Check sheet for the modelled part. Datum: model origin and axes. Units: mm. Face numbers are marked on the shaded views. A direction names the side the tool comes from. Coordinates: 2 decimals unless noted, no trailing zeros. Loops run counter-clockwise (first coordinate to the right, second up) from the corner with the lowest first, then second, coordinate; pieces in that order, holes last.
```python
from build123d import *

# Parameters (mm, degrees)
SKETCH1_R           = 50
BOSS_EXTRUDE1_DEPTH = 35
SKETCH2_R           = 5
BOSS_EXTRUDE2_DEPTH = 45
FILLET1_R           = 10
SKETCH3_R           = 19.698674941
CUT_EXTRUDE1_DEPTH  = 5
SKETCH4_R           = 17.698674941
CUT_EXTRUDE2_DEPTH  = 1
SKETCH5_R           = 15.698674941
CUT_EXTRUDE3_DEPTH  = 1


with BuildPart() as part:
    # Sketch1 → Boss-Extrude1 (new, symmetric)
    with BuildSketch(Plane.XY):
        Circle(SKETCH1_R)
    extrude(amount=BOSS_EXTRUDE1_DEPTH, both=True)

    # Sketch2 → Boss-Extrude2 (add, symmetric)
    with BuildSketch(Plane.XY):
        with Locations(Location((0, 0, 0), (0, 0, 180))):
            Circle(SKETCH2_R)
    extrude(amount=BOSS_EXTRUDE2_DEPTH, both=True)

    # Fillet1
    fillet1_edges = [part.edges().sort_by_distance(p)[0] for p in [
        (-50, 0, -35),
        (-50, 0, 35),
    ]]
    fillet(fillet1_edges, radius=FILLET1_R)

    # Sketch3 → Cut-Extrude1 (cut)
    with BuildSketch(Plane(origin=(50, 0, 0), x_dir=(0, 0, -1), z_dir=(1, 0, 0))):
        Circle(SKETCH3_R)
    extrude(amount=-CUT_EXTRUDE1_DEPTH, mode=Mode.SUBTRACT)

    # Sketch4 → Cut-Extrude2 (cut)
    with BuildSketch(Plane(origin=(45, 0, 0), x_dir=(0, 0, -1), z_dir=(1, 0, 0))):
        Circle(SKETCH4_R)
    extrude(amount=-CUT_EXTRUDE2_DEPTH, mode=Mode.SUBTRACT)

    # Sketch5 → Cut-Extrude3 (cut)
    with BuildSketch(Plane(origin=(44, 0, 0), x_dir=(0, 0, -1), z_dir=(1, 0, 0))):
        Circle(SKETCH5_R)
    extrude(amount=-CUT_EXTRUDE3_DEPTH, mode=Mode.SUBTRACT)


solid = part.part
```
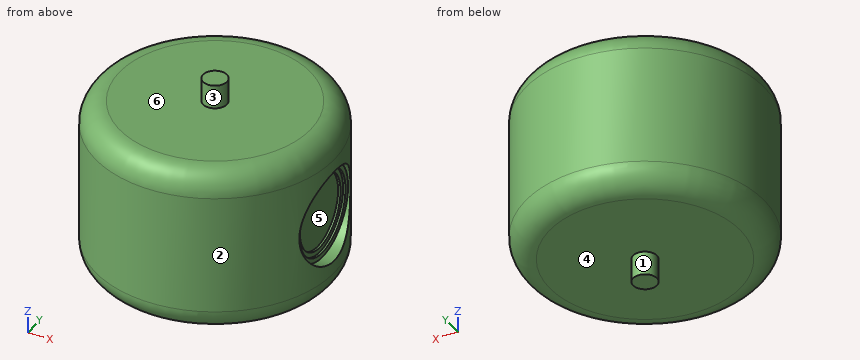
1) Section check C-C on z = 10. Enter the section's corners in (x, y), plus the area to 3 significant figures.
Answer sheet:
outline: (43, -12.1) - (43, 12.1) - (44, 12.1) - (44, 14.6) - (45, 14.6) - (45, 16.97) - (47.03, 16.97) arc R50 ccw (long way) to (47.03, -16.97) - (45, -16.97) - (45, -14.6) - (44, -14.6) - (44, -12.1) - close
area: 7,660 mm2
2) Section check A-A on y = 0. Enter the section's corners in (x, z).
Answer sheet:
outline: (-50, -25) arc R10 ccw to (-40, -35) - (-5, -35) - (-5, -45) - (5, -45) - (5, -35) - (40, -35) arc R10 ccw to (50, -25) - (50, -19.7) - (45, -19.7) - (45, -17.7) - (44, -17.7) - (44, -15.7) - (43, -15.7) - (43, 15.7) - (44, 15.7) - (44, 17.7) - (45, 17.7) - (45, 19.7) - (50, 19.7) - (50, 25) arc R10 ccw to (40, 35) - (5, 35) - (5, 45) - (-5, 45) - (-5, 35) - (-40, 35) arc R10 ccw to (-50, 25) - close
3) Mould release check, pull along Z, two halves, no side actions. Record for the marked faces 3, 4, 5 and 6: +Z half, -Z half, draft (parallel to the pull), parting line (faces both ways), or undercut.
Answer sheet:
face 3: draft
face 4: -Z half
face 5: undercut
face 6: +Z half
4) Section check D-D on z = 0. Enter the section's corners in (x, y).
Answer sheet:
outline: (43, -15.7) - (43, 15.7) - (44, 15.7) - (44, 17.7) - (45, 17.7) - (45, 19.7) - (45.96, 19.7) arc R50 ccw (long way) to (45.96, -19.7) - (45, -19.7) - (45, -17.7) - (44, -17.7) - (44, -15.7) - close
5) Section check B-B on x = 0. Enter the section's corners in (y, z), plus the area to 3 significant figures.
Answer sheet:
outline: (-50, -25) arc R10 ccw to (-40, -35) - (-5, -35) - (-5, -45) - (5, -45) - (5, -35) - (40, -35) arc R10 ccw to (50, -25) - (50, 25) arc R10 ccw to (40, 35) - (5, 35) - (5, 45) - (-5, 45) - (-5, 35) - (-40, 35) arc R10 ccw to (-50, 25) - close
area: 7,110 mm2
6) Depth check by flat-ended pin: pin 1 (5 mm diameter, centred on y = 25.5, z = -19.5, fed in from -X); pin 2 (1 mm diameter, centred on x = 21, y = 27, fed in from -Z); pin 3 (10.5 mm diameter, centred on y = 3.5, z = 5.5, fed in from +X). Enter the tip coordinate at first touch or a pass-through.
Answer sheet:
pin 1: stops at x = -44.4
pin 2: stops at z = -35
pin 3: stops at x = 43
7) Set-up check for the marked faces 1 and 2: record each of +Z, -Z, +X, -X, +Y, -Y from which the full face is reachable in a straight line by a thin tool's end or side.
Answer sheet:
face 1: -Z
face 2: +Z, -Z
8) Scan lines: line 1 (Z direction, x = -20.5, y = 2); line 2 (Y direction, x = 44.75, z = 0); line 3 (Y direction, x = 44.6, z = 0). Record each from-to range of solid material in increasing order.
Answer sheet:
line 1: z = -35 to 35
line 2: y = -22.3 to -17.7, 17.7 to 22.3
line 3: y = -22.6 to -17.7, 17.7 to 22.6
